For this review, take the finished solid that the model builds, in its own axes (mm). Round coordinates to 2 decimals unless told otherwise and drop trailing zeros. Order: outer loops, then holes, each group sorted by start corner. A loop starts at its lowest first (then second) coordinate and runs counter-clockwise, first axis right, second up. Notation, with made-up numbers: M 37,-28 L 72,-28 A26 cw 72,-3 Z; hole C 80,-34.75 d9. An arc over 180 degrees is marked long. Write item = value, one per line. Start each with the question number.
from build123d import *

# Parameters (mm, degrees)
F0_W     = 111.8249478
F0_H     = 357.780717
F0_R     = 1.7272
F1_DEPTH = 3.175
F2_W     = 16.51
F2_H     = 47.9032060428
F3_DEPTH = 3.175


with BuildPart() as f1:
    # F0 (on Top) → F1 (new body)
    with BuildSketch(Plane.XY):
        Rectangle(F0_W, F0_H)
        with Locations((-51.1499739, -174.1278585)):
            Circle(F0_R, mode=Mode.SUBTRACT)
        with Locations((-51.1499739, -155.0778585)):
            Circle(F0_R, mode=Mode.SUBTRACT)
        with Locations((51.1499739, -174.1278585)):
            Circle(F0_R, mode=Mode.SUBTRACT)
        with Locations((51.1499739, -155.0778585)):
            Circle(F0_R, mode=Mode.SUBTRACT)
        with Locations((-51.1499739, 155.0778585)):
            Circle(F0_R, mode=Mode.SUBTRACT)
        with Locations((-51.1499739, 174.1278585)):
            Circle(F0_R, mode=Mode.SUBTRACT)
        with Locations((51.1499739, 155.0778585)):
            Circle(F0_R, mode=Mode.SUBTRACT)
        with Locations((51.1499739, 174.1278585)):
            Circle(F0_R, mode=Mode.SUBTRACT)
    extrude(amount=F1_DEPTH)

    # F2 (on face) → F3 (cut, through all)
    with BuildSketch(Plane.XY.offset(3.175)):
        with Locations((0, -154.9387554786)):
            Rectangle(F2_W, F2_H)
    extrude(amount=-F3_DEPTH, mode=Mode.SUBTRACT)


solid = f1.part
(1) For line 1 along X through (y, z) = (-141.5, 1.75) (3 decimals); line 2 along Y through (x, z) = (2, 0.3), list the stretches that pass through material, from the lowest coordinate up.
(2) We need section B-B, the plane z = 0.6. State how many separate pieces and enclosed holes the cut face has, then the cut area to 3 significant figures.
(3) Insertion check: pin 1 (4 mm diameter, centred on x = 51.15, y = 174.13, fed in from -Z); pin 2 (1 mm diameter, centred on x = 4.5, z = 2, fed in from -Y). Each pin has a flat end and moves straight along its axis. Give the tip position at first contact, or say it passes through.
(4) We need section A-A, the plane y = -139. Write out the cut boundary in (x, z) (3 decimals).
Values:
q1.line_1 = -55.912 to -8.255, 8.255 to 55.912
q1.line_2 = -130.99 to 178.89
q2.separate_pieces = 1
q2.enclosed_holes = 8
q2.area = 39,100 mm²
q3.pin_1 = 0
q3.pin_2 = -130.99
q4.outline = M -55.912,0 L -8.255,0 L -8.255,3.175 L -55.912,3.175 Z; M 8.255,0 L 55.912,0 L 55.912,3.175 L 8.255,3.175 Z
